Model file for the job. Use its own axes, mm. Round coordinates to 2 decimals unless told otherwise and drop trailing zeros. Write each loop counter-clockwise with the first axis right and the second up, starting at its lowest first coordinate (ties: lowest second). Pieces come first, ordered by that corner, then holes. Notation, with made-up numbers: (8.5, -18) - (52.5, -18) arc R27 cw to (52.5, 20) - close; hole circle Ø3 at (47, 40.5). An arc over 180 degrees is marked (long way). Answer as a JSON object with one key per item and string values. Group by question number.
from build123d import *

# Parameters (mm, degrees)
F0_W     = 60.654063
F0_H     = 34.040548
F1_DEPTH = 25.4
F2_SIZE  = 12.7
F4_D     = 6.35


with BuildPart() as f1:
    # F0 (on Front) → F1 (new body)
    with BuildSketch(Plane.XZ):
        with Locations((3.558782, 2.011489)):
            Rectangle(F0_W, F0_H)
    extrude(amount=F1_DEPTH)

    # F2
    f2_edges = [f1.edges().sort_by_distance(p)[0] for p in [
        (3.558783, -25.4, 19.031763),
    ]]
    chamfer(f2_edges, length=F2_SIZE)

    # F4 (through all)
    with Locations(Plane(origin=(0, -15.865882, 15.865882), x_dir=(1, 0, 0), z_dir=(0, -0.707107, 0.707107))):
        with Locations((-13.242152, -4.013676), (17.749857, -3.687446)):
            Hole(F4_D / 2)


solid = f1.part
(1) Slice it at C-C (y = -15.75). Count the separate pieces of the cut face and the enclosed holes in it, then the cut area to 3 significant figures.
(2) Slice it at A-A (x = 10.5). Write the cut outline in (y, z).
(3) Slice it at B-B (x = -15). Write the cut outline in (y, z), then the cut area to 3 significant figures.
(4) Pull direction Z, two halves, no side cores. Call faces 1 (the flat face through (-26.768, -13, 2)), 2 (the flat face through (3.13, -19.14, 12.59)), 3 (the cylindrical face through (-12.55, -10.27, 0.21)): pulls with the +Z half, pulls with the -Z half, needs draft (parallel to the pull), parting line crosses it, or undercut.
(5) Drill centre lines: line 1 (X direction, y = -6, z = -0.5); line 2 (X direction, y = -14.5, z = 6.5); line 3 (Y direction, x = -12, z = 10). Where is each one in solid material? Low to high. Write a range as from..to.
Answer:
{
 "1": {"separate pieces": "1", "enclosed holes": "2", "area": "1,790 mm²"},
 "2": {"outline": "(-25.4, -15.01) - (0, -15.01) - (0, 19.03) - (-12.7, 19.03) - (-25.4, 6.33) - close"},
 "3": {"outline": "(-25.4, -15.01) - (0, -15.01) - (0, -9.42) - (-20.57, 11.16) - (-25.4, 6.33) - close; (-16.83, 14.9) - (0, -1.94) - (0, 19.03) - (-12.7, 19.03) - close", "area": "644 mm²"},
 "4": {"face 1": "needs draft", "face 2": "pulls with the +Z half", "face 3": "undercut"},
 "5": {"line 1": "-26.77..-16.36, -10.12..14.71, 20.79..33.89", "line 2": "-26.77..-15.96, -10.53..15.26, 20.24..33.89", "line 3": "-21.73..-19.81, -11.54..0"}
}
